Model file for the job. Use its own axes, mm. Face numbers are marked on the shaded views. A direction names the side the tool comes from. Coordinates: 2 decimals unless noted, no trailing zeros. Order: outer loops, then holes, each group sorted by start corner. A loop starts at its lowest first (then second) coordinate and runs counter-clockwise, first axis right, second up. Notation, with made-up numbers: (-33, 48.25) -> (-17, 48.25) arc R23 ccw to (-17, 64.25) -> close; hole circle Ø2 at (20.5, 66.5). An arc over 180 degrees is marked (long way). Return JSON: item names as keys, results as strings. Group by question number.
1) Which spindle directions (+Z, -Z, +X, -X, +Y, -Y) get a long thin tool onto all of the face, cutting with end or side? Do the marked faces 5, 6 and 7. Say none if no direction does.
2) Cut at B-B (x = -44). Write the cut outline in (y, z).
3) Cut at A-A (z = -11.5). State how many separate pieces and enclosed holes the cut face has, and give its area (3 significant figures).
4) Flat gauge pins, fed straight in: pin 1 (0.9 mm diameter, centred on y = 10.5, z = -12, fed in from +X); pin 2 (0.6 mm diameter, centred on x = -49, z = -6.5, fed in from +Y); pin 3 (2 mm diameter, centred on x = -39.5, z = -12, fed in from +Y). Where does each tip first touch, or does it go through?
5) Probe line 1 (X direction, y = 10.75, z = -8.75); line 2 (Z direction, x = -51.8, y = 10); line 3 (Z direction, x = -102.5, y = 7.25). List the from-to ranges inside material, lowest first.
6) Pull direction X, two halves, no side cores. Call the marked faces 1, 2, 3 and 4: +X half, -X half, draft (parallel to the pull), parting line (faces both ways), or undercut.
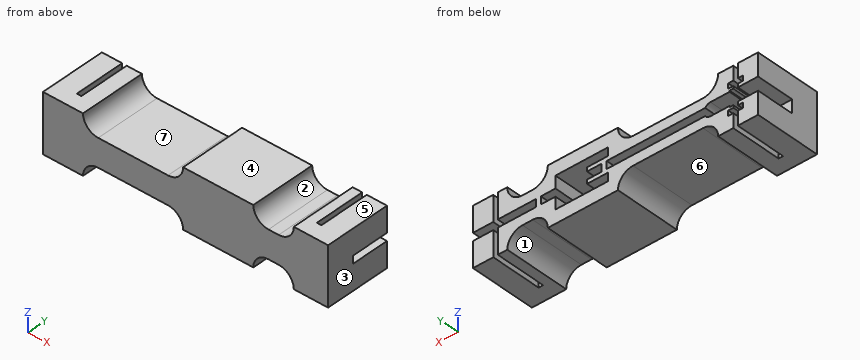
Autodesk Inventor part; units mm, degrees
ref_plane "YZ Plane" through (0, 0, 0) normal (1, 0, 0) x (0, 1, 0)
ref_plane "XZ Plane" through (0, 0, 0) normal (0, 1, 0) x (-1, 0, 0)
ref_plane "XY Plane" through (0, 0, 0) normal (0, 0, 1) x (1, 0, 0)
sketch "Sketch1" plane through (0, 0, 0) normal (0, 1, 0) x (-1, 0, 0)
  line L0 (45.05, -5.25) -> (32.55, -5.25)
  line L1 (32.55, -5.25) -> (32.55, -17.75)
  line L2 (32.55, -17.75) -> (45.05, -17.75)
  line L3 (45.05, -17.75) -> (45.05, -5.25)
  line L4 (0, 0) -> (0, -23)
  line L5 (112.6, -23) -> (112.6, 0)
  line L6 (77.3838, -11.5) -> (49.3838, -11.5) construction
  line L7 (38.8, -2.0322) -> (38.8, -23.0322) construction
  line L8 (93.8, -8.9) -> (112.6, -8.9)
  line L9 (112.6, -14.1) -> (93.8, -14.1)
  line L10 (9.8, 0) -> (9.8, -23)
  line L11 (8, 0) -> (8, -23)
  line L12 (24.8, -10) -> (0, -10)
  line L13 (24.8, -13) -> (0, -13)
  line L14 (102.8, -14.55) -> (101.3, -14.55)
  line L15 (101.3, -14.55) -> (101.3, -8.45)
  line L16 (101.3, -8.45) -> (102.8, -8.45)
  line L17 (50.8, -10) -> (50.8, -13)
  line L18 (50.8, -13) -> (45.05, -13)
  line L19 (45.05, -10) -> (50.8, -10)
  line L20 (32.55, -13) -> (26.8, -13)
  line L21 (26.8, -10) -> (32.55, -10)
  line L22 (102.8, -17.5) -> (100.8, -17.5)
  line L23 (100.8, -17.5) -> (100.8, -15.5)
  line L24 (100.8, -15.5) -> (102.8, -15.5)
  line L25 (102.8, -7.5) -> (100.8, -7.5)
  line L26 (100.8, -7.5) -> (100.8, -5.5)
  line L27 (100.8, -5.5) -> (102.8, -5.5)
  line L28 (137, -16.5) -> (122.5716, -16.5) construction
  line L29 (137, -6.5) -> (123, -6.5) construction
  line L30 (104.6, -17.5) -> (106.6, -17.5)
  line L31 (106.6, -17.5) -> (106.6, -15.5)
  line L32 (106.6, -15.5) -> (104.6, -15.5)
  line L33 (104.6, -7.5) -> (106.6, -7.5)
  line L34 (106.6, -7.5) -> (106.6, -5.5)
  line L35 (106.6, -5.5) -> (104.6, -5.5)
  line L36 (104.6, -23) -> (104.6, -17.5)
  line L37 (102.8, -17.5) -> (102.8, -23)
  line L38 (104.6, -15.5) -> (104.6, -7.5)
  line L39 (104.6, -5.5) -> (104.6, 0)
  line L40 (102.8, 0) -> (102.8, -5.5)
  line L41 (102.8, -7.5) -> (102.8, -15.5)
  line L42 (45.05, -17.75) -> (53.25, -17.75)
  line L43 (53.25, -17.75) -> (53.25, -14.55)
  line L44 (53.25, -14.55) -> (45.05, -14.55)
  line L45 (45.05, -8.45) -> (53.25, -8.45)
  line L46 (53.25, -8.45) -> (53.25, -5.25)
  line L47 (53.25, -5.25) -> (45.05, -5.25)
  line L48 (48.05, -17.75) -> (48.05, -14.55)
  line L49 (50.05, -17.75) -> (50.05, -14.55)
  line L50 (50.05, -8.45) -> (50.05, -5.25)
  line L51 (48.05, -8.45) -> (48.05, -5.25)
  line L52 (52.8, -10) -> (52.8, -13)
  line L53 (26.8, -10) -> (26.8, -13)
  line L54 (24.8, -10) -> (24.8, -13)
  line L55 (52.8, -13) -> (91.6763, -13)
  line L56 (52.8, -10) -> (91.6763, -10)
  arc A0 (93.8, -8.9) -> (91.6763, -10) centre (93.8, -11.5) ccw
  arc A1 (91.6763, -13) -> (93.8, -14.1) centre (93.8, -11.5) ccw
  arc A2 (96.8, -23) -> (90.8, -17) centre (90.8, -23) ccw
  arc A3 (63.25, -17) -> (57.25, -23) centre (63.25, -23) ccw
  arc A4 (90.8, -6) -> (96.8, 0) centre (90.8, 0) ccw
  arc A5 (57.25, 0) -> (63.25, -6) centre (63.25, 0) ccw
  line L57 (90.8, -17) -> (63.25, -17)
  line L58 (90.8, -6) -> (63.25, -6)
  line L59 (112.6, 0) -> (96.8, 0)
  line L60 (96.8, -23) -> (112.6, -23)
  arc A6 (29.55, -23) -> (23.55, -17) centre (23.55, -23) ccw
  arc A7 (23.55, -6) -> (29.55, 0) centre (23.55, 0) ccw
  arc A8 (19.55, -17) -> (13.55, -23) centre (19.55, -23) ccw
  arc A9 (13.55, 0) -> (19.55, -6) centre (19.55, 0) ccw
  line L61 (23.55, -6) -> (19.55, -6)
  line L62 (23.55, -17) -> (19.55, -17)
  line L63 (0, -23) -> (13.55, -23)
  line L64 (29.55, -23) -> (57.25, -23)
  line L65 (57.25, 0) -> (29.55, 0)
  line L66 (13.55, 0) -> (0, 0)
  line L67 (115.3, -25) -> (115.3, 2)
  line L68 (-2.7, 2) -> (-2.7, -25)
  arc A10 (65.25, -19) -> (59.25, -25) centre (65.25, -25) ccw
  arc A11 (94.8, -25) -> (88.8, -19) centre (88.8, -25) ccw
  line L69 (56.3, -20.25) -> (56.3, -1) construction
  arc A12 (59.25, 2) -> (65.25, -4) centre (65.25, 2) ccw
  arc A13 (88.8, -4) -> (94.8, 2) centre (88.8, 2) ccw
  arc A14 (15.55, 2) -> (27.55, 2) centre (21.55, 2) ccw
  arc A15 (27.55, -25) -> (15.55, -25) centre (21.55, -25) ccw
  line L70 (88.8, -19) -> (65.25, -19)
  line L71 (88.8, -4) -> (65.25, -4)
  line L72 (115.3, 2) -> (94.8, 2)
  line L73 (94.8, -25) -> (115.3, -25)
  line L74 (-2.7, -25) -> (15.55, -25)
  line L75 (27.55, -25) -> (59.25, -25)
  line L76 (59.25, 2) -> (27.55, 2)
  line L77 (15.55, 2) -> (-2.7, 2)
  line L78 (125.6323, 7.0516) -> (125.6323, -28.0034) construction
  line L79 (125.6323, -28.0034) -> (118.769, -28.0034) construction
  line L80 (118.769, -28.0034) -> (118.769, 7.0516) construction
  line L81 (118.769, 7.0516) -> (125.6323, 7.0516) construction
  point P0 (104.6, -8.9)
  point P1 (104.6, -14.1)
  point P2 (102.8, -8.9)
  point P3 (102.8, -14.1)
  point P4 (9.8, -13)
  point P5 (8, -13)
  point P6 (8, -10)
  point P7 (9.8, -10)
  point P8 (38.8, -11.5)
  point P9 (101.3, -14.1)
  point P10 (101.3, -8.9)
  dimension "d0" = 12.5
  dimension "d1" = 12.5
  dimension "d3" = 23
  dimension "d12" = 5.2
  dimension "d20" = 1.8
  dimension "d25" = 3
  dimension "d36" = 6.1
  dimension "d37" = 1.5
  dimension "d62" = 3
  dimension "d63" = 3
  dimension "d94" = 2
  dimension "d95" = 2
  dimension "d96" = 10
  dimension "d97" = 1.8
  dimension "d106" = 8.2
  dimension "d107" = 3
  dimension "d108" = 2
  dimension "d109" = 3.2
  dimension "d113" = 1.5
  dimension "d114" = 2
  dimension "d115" = 64
  dimension "d116" = 29
  dimension "d117" = 8
  dimension "d118" = 8
  dimension "d119" = 2
  dimension "d120" = 12
  dimension "d121" = 12
  dimension "d122" = 9
  dimension "d129" = 12
  dimension "d130" = 12
  dimension "d131" = 10
  dimension "d134" = 9
  dimension "d135" = 4
  dimension "d149" = 118
  dimension "d150" = 27
  dimension "d152" = 11
  dimension "d153" = 12
  dimension "d154" = 14
extrude "Extrusion16" add sketch "Sketch1" against normal blind 6 contours L3 L2 L1 L0 | L47 L51 L45 L3 | L47 L50 L45 L51 | L1 L20 L53 L21 | L19 L17 L18 L3 | L47 L46 L45 L50 | L44 L48 L42 L3 | L44 L49 L42 L48 | L44 L43 L42 L49 | L66 L11 L12 L4 | L12 L11 L13 L4 | L66 L10 L12 L11 | L13 L11 L63 L4 | L12 L10 L13 L11 | L66 A9 L61 A7 L65 A5 L58 A4 L59 L40 L27 L26 L25 L41 L16 L15 L8 A0 L56 L52 L55 A1 L9 L14 L24 L23 L22 L37 L60 A2 L57 A3 L64 A6 L62 A8 L63 L10 L13 L54 L12 | L13 L10 L63 L11 | L12 L54 L13 L10 | L59 L39 L35 L34 L33 L38 L8 L41 L25 L26 L27 L40 | L59 L5 L8 L38 L33 L34 L35 L39 | L37 L22 L23 L24 L41 L9 L38 L32 L31 L30 L36 L60 | L5 L9 L38 L8 | L36 L30 L31 L32 L38 L9 L5 L60 | L38 L9 L41 L8 | L41 L8 L15 L16 | L41 L9 L15 L8 | L41 L14 L15 L9 | L15 L9 A1 L55 L52 L56 A0 L8
extrude "Extrusion17" add sketch "Sketch1" along normal blind 20 contours L66 L11 L12 L4 | L13 L11 L63 L4 | L66 A9 L61 A7 L65 A5 L58 A4 L59 L40 L27 L26 L25 L41 L16 L15 L8 A0 L56 L52 L55 A1 L9 L14 L24 L23 L22 L37 L60 A2 L57 A3 L64 A6 L62 A8 L63 L10 L13 L54 L12 | L59 L5 L8 L38 L33 L34 L35 L39 | L36 L30 L31 L32 L38 L9 L5 L60
extrude "Extrusion18" add sketch "Sketch1" along normal blind 5 contours L1 L20 L53 L21 | L19 L17 L18 L3 | L12 L11 L13 L4 | L12 L54 L13 L10 | L5 L9 L38 L8 | L15 L9 A1 L55 L52 L56 A0 L8
extrude "Extrusion19" add sketch "Sketch1" along normal blind 9 contours L47 L50 L45 L51 | L44 L49 L42 L48
sketch "Sketch2" plane through (0, -6, 0) normal (1, 0, 0) x (0, 0, -1)
  line L0 (11.5, 16) -> (11.5, 6.397) construction
  line L1 (0, 6) -> (23, 6) construction
  line L2 (0, 1.5617) -> (0, -5) construction
  line L3 (23, -1.6862) -> (23, -8) construction
  point P0 (11.5, 16)
  dimension "d139" = 10
hole "Hole1" at (0, 10, -11.5) direction (-1, 0, 0) diameter 2 end through all
properties part number "Spirulina_prototype2"
Answers below:
{
 "1": {"face 5": "+Z, +X, -X, +Y, -Y", "face 6": "-Z, +Y, -Y", "face 7": "+Z, +Y, -Y"},
 "2": {"outline": "(-6, -23) -> (20, -23) -> (20, -17.75) -> (0, -17.75) -> (0, -5.25) -> (20, -5.25) -> (20, 0) -> (-6, 0) -> close"},
 "3": {"separate pieces": "3", "enclosed holes": "0", "area": "1,200 mm^2"},
 "4": {"pin 1": "stops at x = -24.8", "pin 2": "stops at y = 9", "pin 3": "stops at y = 0"},
 "5": {"line 1": "x = -112.6 to -104.6, -101.3 to -45.05, -32.55 to -9.8, -8 to 0", "line 2": "z = -23 to -17.75, -14.55 to -12.5, -10.5 to -8.45, -5.25 to 0", "line 3": "z = -23 to -17.5, -15.5 to -14.55, -8.45 to -7.5, -5.5 to 0"},
 "6": {"face 1": "undercut", "face 2": "undercut", "face 3": "+X half", "face 4": "draft"}
}
